Geometry: see drawing. Coordinates: mm, zero at the bounding-box minimum. Give positions to 0.01 mm unless a question says otherwise; leave off trailing zeros. Write each loop counter-clockwise with the first axis right and the second up, starting at its lowest first coordinate (ties: lowest second). Pieces come first, ordered by that corner, then holes. Notation, with made-up numbers: (69.5, 75) -> (108.5, 75) arc R20 ccw to (108.5, 103) -> close; hole circle Ø7 at (83, 48.25). An arc over 180 degrees is marked (long way). Use one line per item in the form item = value. Start each with the question number.
(1) First-contact query: P1, Ø6, axis at x = 12, z = 5.5, coming from the +Y side. Flat tip, straight axial feed; report the tip coordinate or a pass-through.
(2) Draft query along X for the marked faces 1 and 2. Return one class per face: pulls with the +X half, pulls with the -X half, needs draft (parallel to the pull), parting line crosses it, or undercut.
(3) Material intervals for line 1 along X through (y, z) = (2.05, 24); line 2 along Y through (x, z) = (18, 7.25), sorted ascending. Write a range as from..to.
(4) Cut plane B-B, the plane z = 20.75. Output: boundary loops of the cut face in (x, y).
(5) Cut plane A-A, the plane y = 2.65. Output: boundary loops of the cut face in (x, z), and give its area (3 significant figures).
(6) Cut plane C-C, the plane x = 36. Output: boundary loops of the cut face in (y, z).
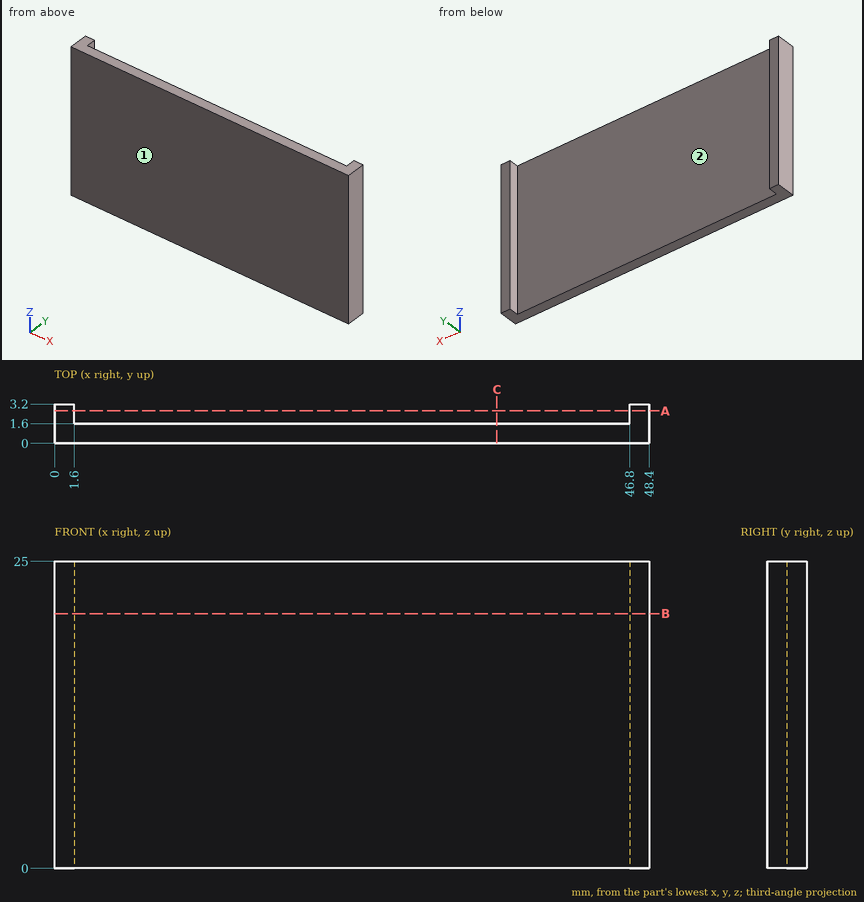
Geometry says:
q1.P1 = 1.6
q2.face_1 = needs draft
q2.face_2 = undercut
q3.line_1 = 0..1.6, 46.8..48.4
q3.line_2 = 0..1.6
q4.outline = (0, 0) -> (48.4, 0) -> (48.4, 3.2) -> (46.8, 3.2) -> (46.8, 1.6) -> (1.6, 1.6) -> (1.6, 3.2) -> (0, 3.2) -> close
q5.outline = (0, 0) -> (1.6, 0) -> (1.6, 25) -> (0, 25) -> close; (46.8, 0) -> (48.4, 0) -> (48.4, 25) -> (46.8, 25) -> close
q5.area = 80.0 mm^2
q6.outline = (0, 0) -> (1.6, 0) -> (1.6, 25) -> (0, 25) -> close
